Geometry: final body of the model. Coordinates: model frame, mm. Face numbers are marked on the shaded views. Round coordinates to 2 decimals unless told otherwise and drop trailing zeros. Loops run counter-clockwise (first coordinate to the right, second up) from the corner with the lowest first, then second, coordinate; pieces in that order, holes last. Notation, with made-up numbers: M -28,36.25 L -2,36.25 A29 ccw -2,64.25 Z; hole C 85.5,51 d1. An arc over 180 degrees is marked long. Write each question's results on one line, items separated by ' | '.
```python
from build123d import *

# Parameters (mm, degrees)
SKETCH1_R           = 40
SKETCH1_R_2         = 25.25
SKETCH1_R_3         = 3.25
BOSS_EXTRUDE1_DEPTH = 6


with BuildPart() as part:
    # Sketch1 → Boss-Extrude1 (new body, symmetric)
    with BuildSketch(Plane.XY):
        Circle(SKETCH1_R)
        Circle(SKETCH1_R_2, mode=Mode.SUBTRACT)
        with Locations((-32.5, 0)):
            Circle(SKETCH1_R_3, mode=Mode.SUBTRACT)
        with Locations((0, 32.5)):
            Circle(SKETCH1_R_3, mode=Mode.SUBTRACT)
        with Locations((0, -32.5)):
            Circle(SKETCH1_R_3, mode=Mode.SUBTRACT)
        with Locations((32.5, 0)):
            Circle(SKETCH1_R_3, mode=Mode.SUBTRACT)
    extrude(amount=BOSS_EXTRUDE1_DEPTH, both=True)


solid = part.part
```
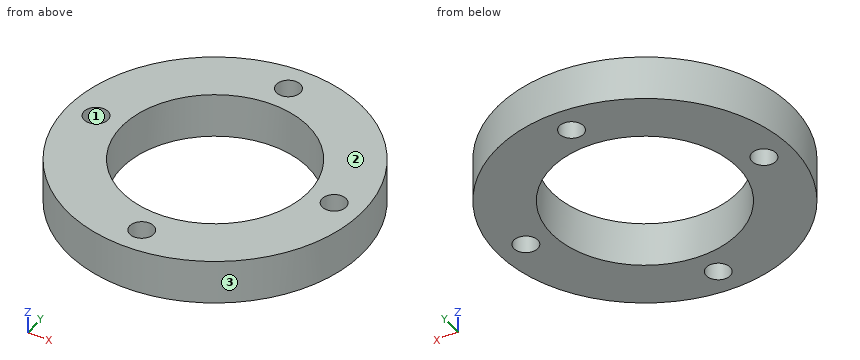
1. Pin query (flat end, axial travel): P1, Ø1.5, axis at x = 1, z = 1.5, coming from the +Y side; P2, Ø6, axis at y = -29, z = 3, coming from the +X side. Return the tip coordinate at first contact, or that it passes through.
Answer key:
P1: stops at y = 40 | P2: stops at x = 30.4
2. Ray query, probe 1 along Y at (x, z) = (0, -2.5); probe 2 along X at (y, z) = (17, 0); probe 3 along Y at (x, z) = (32.5, -1). Return the intervals inside material, ascending.
Answer key:
probe 1: y = -40 to -35.75, -29.25 to -25.25, 25.25 to 29.25, 35.75 to 40 | probe 2: x = -36.21 to -18.67, 18.67 to 36.21 | probe 3: y = -23.32 to -3.25, 3.25 to 23.32
3. Section C-C (z = 3.75). Output: boundary loops of the cut face in (x, y), then the cut area to 3 significant figures.
Answer key:
outline: C 0,0 d80; hole C -32.5,0 d6.5; hole C 0,0 d50.5; hole C 0,-32.5 d6.5; hole C 0,32.5 d6.5; hole C 32.5,0 d6.5 | area: 2,890 mm²
4. Section D-D (x = 32.5). Output: boundary loops of the cut face in (y, z), then the cut area to 3 significant figures.
Answer key:
outline: M -23.32,-6 L -3.25,-6 L -3.25,6 L -23.32,6 Z; M 3.25,-6 L 23.32,-6 L 23.32,6 L 3.25,6 Z | area: 482 mm²
5. Section A-A (y = 0). Output: boundary loops of the cut face in (x, z), then the cut area to 3 significant figures.
Answer key:
outline: M -40,-6 L -35.75,-6 L -35.75,6 L -40,6 Z; M -29.25,-6 L -25.25,-6 L -25.25,6 L -29.25,6 Z; M 25.25,-6 L 29.25,-6 L 29.25,6 L 25.25,6 Z; M 35.75,-6 L 40,-6 L 40,6 L 35.75,6 Z | area: 198 mm²
6. Draft query along Y for the marked faces 1, 2 and 3. Return one class per face: pulls with the +Y half, pulls with the -Y half, needs draft (parallel to the pull), parting line crosses it, or undercut.
Answer key:
face 1: undercut | face 2: needs draft | face 3: parting line crosses it
